Read the model definition and answer for the solid it produces. Units are mm, in the model's axes. Face numbers are marked on the shaded views. A direction names the side the tool comes from. Coordinates: 2 decimals unless noted, no trailing zeros. Write each loop counter-clockwise with the first axis right and the second up, starting at its lowest first coordinate (ties: lowest second). Pieces come first, ordered by that corner, then holes.
(1) Section B-B on x = 0 is taken. Write down the section's boundary in (y, z).
(2) Section D-D on x = -3.5 is taken. Write down the section's boundary in (y, z), then the cut area to 3 significant figures.
(3) Section C-C on y = 0.5 is taken. Write down the section's boundary in (x, z).
(4) The mould has two halves that part along X. Classify the marked faces 3, 4 and 5: +X half, -X half, draft (parallel to the pull), parting line (faces both ways), or undercut.
(5) Section A-A on z = 0 is taken. Write down the section's boundary in (x, y), then the cut area to 4 significant figures.
(6) Given pin 1 (4 mm diameter, centred on x = 2, z = 3, fed in from +Y), flat-ended and moving along its own axis, determine where the tip first touches the part or whether it passes through.
(7) Which of the six approach directions +Z, -Z, +X, -X, +Y, -Y give full straight-line access (tool end or side, diameter ignored) to the marked faces 1 and 2?
(8) Find the intervals of material crossed by probe 1 along Z at (x, y) = (0, 3); probe 2 along Y at (x, z) = (-2, 6); probe 3 along X at (y, z) = (2, 7.5), in increasing order.
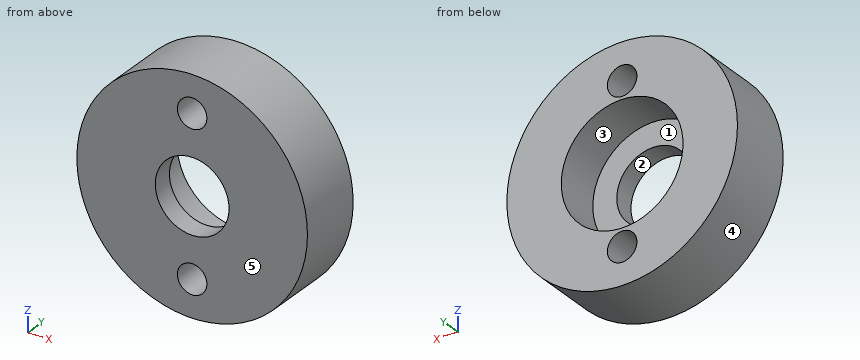
Autodesk Inventor part; units mm, degrees
ref_plane "YZ Plane" through (0, 0, 0) normal (1, 0, 0) x (0, 1, 0)
ref_plane "XZ Plane" through (0, 0, 0) normal (0, 1, 0) x (-1, 0, 0)
ref_plane "XY Plane" through (0, 0, 0) normal (0, 0, 1) x (1, 0, 0)
sketch "草圖1" plane through (0, 0, 0) normal (0, 1, 0) x (-1, 0, 0)
  circle A0 centre (0, 0) radius 12.5
  circle A1 centre (0, 8.5) radius 1.6
  circle A2 centre (0, -8.5) radius 1.6
  dimension "d0" = 25
  dimension "d1" = 17
  dimension "d2" = 8.5
  dimension "d3" = 3.2
  dimension "d4" = 3.2
extrude "擠出1" add sketch "草圖1" along normal blind 6
sketch "草圖2" plane through (0, 6, 0) normal (0, 1, 0) x (1, 0, 0)
  circle A0 centre (0, 0) radius 4
  dimension "d7" = 8
extrude "擠出2" cut sketch "草圖2" against normal through all
sketch "草圖3" plane through (0, 6, 0) normal (0, 1, 0) x (1, 0, 0)
  circle A0 centre (0, 0) radius 6.6
  dimension "d10" = 13.2
extrude "擠出3" cut sketch "草圖3" against normal blind 5
move faces "移動1" translate (0, -1.25, 0) faces at (3.5966, 0, -7.1119)
equation "\"d4\" = d3"
properties part number "wheel_base_cover_print"
Response:
1. outline: (-1.25, -12.5) - (6, -12.5) - (6, -10.1) - (-1.25, -10.1) - close; (-1.25, -6.9) - (6, -6.9) - (6, -6.6) - (1, -6.6) - (1, -4) - (-1.25, -4) - close; (-1.25, 4) - (1, 4) - (1, 6.6) - (6, 6.6) - (6, 6.9) - (-1.25, 6.9) - close; (-1.25, 10.1) - (6, 10.1) - (6, 12.5) - (-1.25, 12.5) - close
2. outline: (-1.25, -12) - (6, -12) - (6, -5.6) - (1, -5.6) - (1, -1.94) - (-1.25, -1.94) - close; (-1.25, 1.94) - (1, 1.94) - (1, 5.6) - (6, 5.6) - (6, 12) - (-1.25, 12) - close
2. area: 109 mm2
3. outline: circle Ø25 at (0, 0); hole circle Ø8 at (0, 0); hole circle Ø3.2 at (0, -8.5); hole circle Ø3.2 at (0, 8.5)
4. face 3: undercut
4. face 4: parting line
4. face 5: draft
5. outline: (-12.5, -1.25) - (-4, -1.25) - (-4, 1) - (-6.6, 1) - (-6.6, 6) - (-12.5, 6) - close; (4, -1.25) - (12.5, -1.25) - (12.5, 6) - (6.6, 6) - (6.6, 1) - (4, 1) - close
5. area: 97.25 mm2
6. pin 1: stops at y = 1
7. face 1: +Y
7. face 2: +Y, -Y
8. probe 1: z = -12.5 to -10.1, -6.9 to -6.6, 6.6 to 6.9, 10.1 to 12.5
8. probe 2: y = -1.25 to 1
8. probe 3: x = -10 to -1.25, 1.25 to 10
